from build123d import *

# Parameters (mm, degrees)
PLAT_W                      = 30
PLAT_H                      = 5
EL_MENT_M_CANO_SOUD_1_DEPTH = 385
ESQUISSE2_R                 = 8
ENL_V_MAT_EXTRU_1_DEPTH     = 10
ESQUISSE3_W                 = 80
ESQUISSE3_H                 = 8
ENL_V_MAT_EXTRU_2_DEPTH     = 10
CONG_1_R                    = 4
ESQUISSE4_R                 = 4
ENL_V_MAT_EXTRU_3_DEPTH     = 10
R_P_TITION_LIN_AIRE1_COUNT  = 9
R_P_TITION_LIN_AIRE1_PITCH  = 9
CONG_2_R                    = 4


with BuildPart() as part:
    # plat → Elément mécano-soudé1 (new body)
    with BuildSketch(Plane.YZ.offset(-192.5)):
        Rectangle(PLAT_W, PLAT_H)
    extrude(amount=EL_MENT_M_CANO_SOUD_1_DEPTH)

    # Esquisse2 → Enlèv. mat.-Extru.1 (cut)
    with BuildSketch(Plane.XY.offset(2.5)):
        with Locations((-176.5, 0)):
            Circle(ESQUISSE2_R)
    extrude(amount=-ENL_V_MAT_EXTRU_1_DEPTH, mode=Mode.SUBTRACT)

    # Esquisse3 → Enlèv. mat.-Extru.2 (cut)
    with BuildSketch(Plane.XY.offset(2.5)):
        with Locations((-82.5, -2)):
            Rectangle(ESQUISSE3_W, ESQUISSE3_H)
    extrude(amount=-ENL_V_MAT_EXTRU_2_DEPTH, mode=Mode.SUBTRACT)

    # Congé1
    cong_1_edges = [part.edges().sort_by_distance(p)[0] for p in [
        (-42.5, 2, 0),
        (-122.5, 2, 0),
    ]]
    fillet(cong_1_edges, radius=CONG_1_R)

    # Esquisse4 → Enlèv. mat.-Extru.3 (cut)
    with BuildSketch(Plane.XY.offset(2.5)):
        with Locations((-118.5, -6)):
            Circle(ESQUISSE4_R)
    enl_v_mat_extru_3 = extrude(amount=-ENL_V_MAT_EXTRU_3_DEPTH, mode=Mode.SUBTRACT)

    # Répétition linéaire1: Enlèv. mat.-Extru.3 ×9
    with Locations(*[(i * R_P_TITION_LIN_AIRE1_PITCH, 0, 0) for i in range(1, R_P_TITION_LIN_AIRE1_COUNT)]):
        add(enl_v_mat_extru_3, mode=Mode.SUBTRACT)

    # Congé2
    cong_2_edges = [part.edges().sort_by_distance(p)[0] for p in [
        (192.5, 15, 0),
        (192.5, -15, 0),
        (-192.5, 15, 0),
        (-192.5, -15, 0),
    ]]
    fillet(cong_2_edges, radius=CONG_2_R)


solid = part.part
Model file for the job. Use its own axes, mm. Give positions to 0.01 mm unless a question says otherwise; leave off trailing zeros. Loops run counter-clockwise (first coordinate to the right, second up) from the corner with the lowest first, then second, coordinate; pieces in that order, holes last. Notation, with made-up numbers: (84, 40.5) - (108, 40.5) arc R10 cw to (108, 59.5) - close; hole circle Ø8 at (27, -35.75). An arc over 180 degrees is marked (long way). Use one line per item in the form item = value.
(1) Cut at C-C (x = -176.5). Give the cut face in (y, z), then the cut area to 3 significant figures.
Determined:
outline = (-15, -2.5) - (-8, -2.5) - (-8, 2.5) - (-15, 2.5) - close; (8, -2.5) - (15, -2.5) - (15, 2.5) - (8, 2.5) - close
area = 70.0 mm^2
(2) Cut at A-A (x = -82.5). Give the cut face in (y, z), then the cut area to 3 significant figures.
Determined:
outline = (-15, -2.5) - (-10, -2.5) - (-10, 2.5) - (-15, 2.5) - close; (2, -2.5) - (15, -2.5) - (15, 2.5) - (2, 2.5) - close
area = 90.0 mm^2
(3) Pull direction Y, two halves, no side cores. Call faces 1 (the face through (-184.492, 0.352, 0.035)), 2 (the face through (-3, 0, 2.5)): pulls with the +Y half, pulls with the -Y half, needs draft (parallel to the pull), parting line crosses it, or undercut.
Determined:
face_1 = undercut
face_2 = needs draft
(4) Cut at B-B (z = 0.7). Count the separate pieces of the cut face and the enclosed holes in it, then the cut area to 3 significant figures.
Determined:
separate_pieces = 1
enclosed_holes = 2
area = 10,500 mm^2
(5) Drill centre lines: L1, parallel to Y at x = -176.5, z = 0.95; L2, parallel to X at y = -11.5, z = -1.15; L3, parallel to X at y = -1.5, z = 1.05. Where is each one in solid material? Low to high.
Determined:
L1 = -15 to -8, 8 to 15
L2 = -192.47 to 192.47
L3 = -192.5 to -184.36, -168.64 to -122.47, -42.53 to 192.5
